Autodesk Inventor part; units mm, degrees
ref_plane "YZ Plane" through (0, 0, 0) normal (1, 0, 0) x (0, 1, 0)
ref_plane "XZ Plane" through (0, 0, 0) normal (0, 1, 0) x (-1, 0, 0)
ref_plane "XY Plane" through (0, 0, 0) normal (0, 0, 1) x (1, 0, 0)
sketch "Sketch1" plane through (0, 0, 0) normal (0, 0, 1) x (1, 0, 0)
  line L0 (-85, 15) -> (85, 15)
  line L1 (85, 15) -> (85, -15)
  line L2 (85, -15) -> (-85, -15)
  line L3 (-85, -15) -> (-85, 15)
  line L4 (85, -15) -> (-85, -15)
  line L5 (-85, -15) -> (-85, -23.1)
  line L6 (-85, -23.1) -> (85, -23.1)
  line L7 (85, -23.1) -> (85, -15)
  point P0 (0, 0)
  dimension "d0" = 30
  dimension "d1" = 170
  dimension "d2" = 85
  dimension "d3" = 15
  dimension "d34" = 8.1
  dimension "d35" = 170
extrude "Extrusion1" add sketch "Sketch1" along normal blind 10
sketch "Sketch2" plane through (0, 0, 10) normal (0, 0, 1) x (1, 0, 0)
  point P0 (0, 0)
  point P1 (-37.5, 0)
  point P2 (-12.5, 0)
  point P3 (12.5, 0)
  point P4 (37.5, 0)
  dimension "d30" = 25
  dimension "d31" = 25
  dimension "d32" = 25
  dimension "d33" = 12.5
hole "Hole1" at (-37.5, 0, 10) at (-12.5, 0, 10) at (12.5, 0, 10) at (37.5, 0, 10) direction (0, 0, -1) diameter 6.6 end through all counterbore diameter 11 counterbore depth 7
sketch "Sketch3" plane through (0, 0, 10) normal (0, 0, 1) x (1, 0, 0)
  point P0 (0, 0)
  point P1 (75, 0)
  point P2 (-75, 0)
  dimension "d16" = 150
  dimension "d17" = 75
hole "Hole2" at (75, 0, 10) at (-75, 0, 10) direction (0, 0, -1) diameter 3.242 end through all
equation "\"d35\" = d1"
properties part number "zStackJackAttach_piece2"
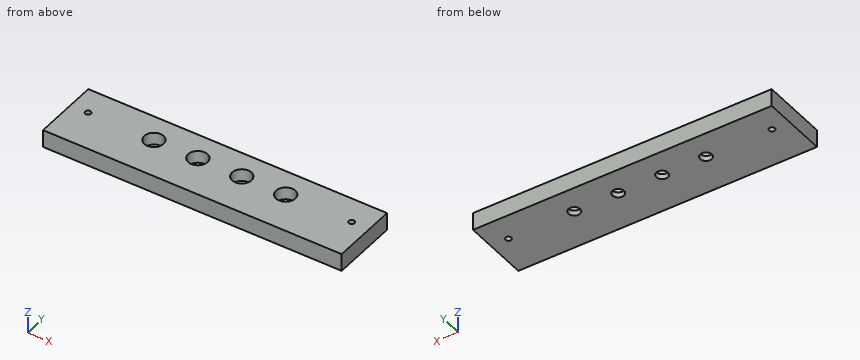
Geometry: final body of the model. Coordinates: model frame, mm. Coordinates: 2 decimals unless noted, no trailing zeros. Order: outer loops, then holes, each group sorted by start corner. A loop starts at its lowest first (then second) coordinate and runs counter-clockwise, first axis right, second up. Notation, with made-up numbers: (-38, -11.75) - (1, -11.75) arc R24 ccw to (1, 22.25) - close; hole circle Ø5 at (53.25, 32.25). An arc over 180 degrees is marked (long way). Return JSON: item names as keys, results as strings. Group by question number.
1. Material intervals for line 1 along Y through (x, z) = (12.5, 5.75); line 2 along Y through (x, z) = (75, 4.5); line 3 along X through (y, z) = (-5, 4), sorted ascending. Write a range as [from, to].
2. Pin query (flat end, axial travel): pin 1 (4 mm diameter, centred on x = 12.5, y = 0, fed in from -Z); pin 2 (12 mm diameter, centred on x = -38, y = 0, fed in from +Z); pin 3 (8.5 mm diameter, centred on x = -37.5, y = 0, fed in from +Z). Return the tip coordinate at first contact, or that it passes through.
3. Cut plane B-B (z = 6.75). Output: boundary loops of the cut face in (x, y), plus the area to 3 significant figures.
4. Cut plane C-C (x = -12.5). Output: boundary loops of the cut face in (y, z), plus the area to 3 significant figures.
5. Cut plane A-A (x = 75). Output: boundary loops of the cut face in (y, z), plus the area to 3 significant figures.
6. Cut plane D-D (x = 39). Output: boundary loops of the cut face in (y, z), plus the area to 3 significant figures.
Resolved:
{
 "1": {"line 1": "y = [-23.1, -5.5], [5.5, 15]", "line 2": "y = [-23.1, -1.62], [1.62, 15]", "line 3": "x = [-85, -39.79], [-35.21, -14.79], [-10.21, 10.21], [14.79, 35.21], [39.79, 85]"},
 "2": {"pin 1": "passes through", "pin 2": "stops at z = 10", "pin 3": "stops at z = 3"},
 "3": {"outline": "(-85, -23.1) - (85, -23.1) - (85, 15) - (-85, 15) - close; hole circle Ø3.24 at (-75, 0); hole circle Ø11 at (-37.5, 0); hole circle Ø11 at (-12.5, 0); hole circle Ø11 at (12.5, 0); hole circle Ø11 at (37.5, 0); hole circle Ø3.24 at (75, 0)", "area": "6,080 mm²"},
 "4": {"outline": "(-23.1, 0) - (-3.3, 0) - (-3.3, 3) - (-5.5, 3) - (-5.5, 10) - (-23.1, 10) - close; (3.3, 0) - (15, 0) - (15, 10) - (5.5, 10) - (5.5, 3) - (3.3, 3) - close", "area": "284 mm²"},
 "5": {"outline": "(-23.1, 0) - (-1.62, 0) - (-1.62, 10) - (-23.1, 10) - close; (1.62, 0) - (15, 0) - (15, 10) - (1.62, 10) - close", "area": "349 mm²"},
 "6": {"outline": "(-23.1, 0) - (-2.94, 0) - (-2.94, 3) - (-5.29, 3) - (-5.29, 10) - (-23.1, 10) - close; (2.94, 0) - (15, 0) - (15, 10) - (5.29, 10) - (5.29, 3) - (2.94, 3) - close", "area": "289 mm²"}
}
